Could you check a few things on this drawing? It's one solid part, dimensions in mm from its lowest x, y, z. Give positions to 0.01 mm unless a question says otherwise; leave off trailing zeros. Write each loop counter-clockwise with the first axis right and the second up, starting at its lowest first coordinate (ties: lowest second). Pieces come first, ordered by that corner, then holes. Notation, with made-up numbers: (49.5, 45.5) -> (72.5, 45.5) arc R19 ccw to (72.5, 80.5) -> close; hole circle Ø8 at (10.25, 75.5). An arc over 180 degrees is marked (long way). Answer as CSV lines item,"result". Start each with the question number.
1. If we section it at D-D on z = 8.5: Write out the boundary of the cut face in (x, y) (1 decimal), plus the area to 3 significant figures.
2. I'm going to push flat-ended pins straight in: P1, Ø1.5, axis at x = 18.5, y = 2.5, coming from the +Z side; P2, Ø1.5, axis at x = 14.5, y = 2, coming from the -Z side. Where does each tip first touch, or does it pass through?
3. If we section it at B-B on z = 34: Write out the boundary of the cut face in (x, y) (1 decimal).
4. I need wall thicknesses on line 1 (X direction, y = 1.75, z = 18.5) (1 decimal); line 2 (X direction, y = 4.45, z = 32); line 3 (Y direction, x = 3.5, z = 32.5) (1 decimal). Which ranges of each line are inside material? Lowest first, please. Write a range as [from, to].
5. If we mould it in two halves opening along X, with no side actions, what happens to the marked faces 1, 2, 3 and 4? For each: pulls with the +X half, pulls with the -X half, needs draft (parallel to the pull), parting line crosses it, or undercut.
6. If we section it at A-A on y = 2.5: Count the separate pieces of the cut face and the enclosed holes in it.
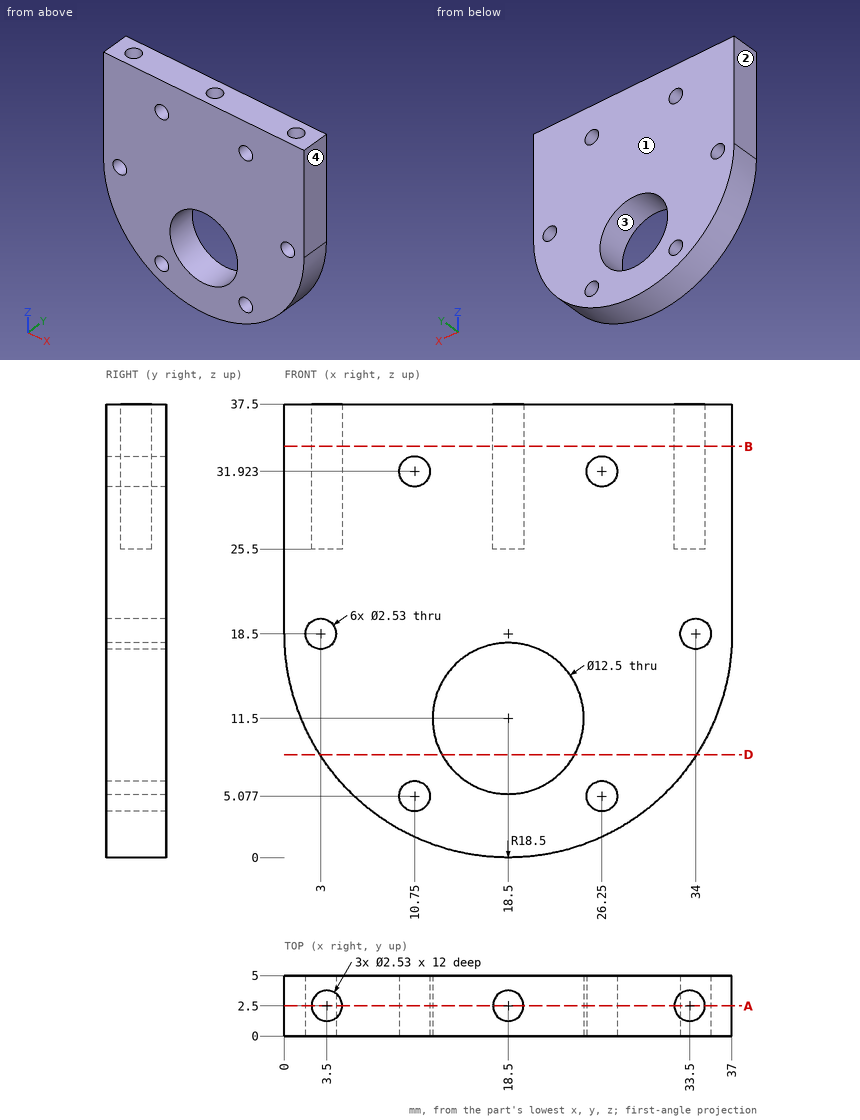
Computed values:
1,outline,"(2.9, 0) -> (13, 0) -> (13, 5) -> (2.9, 5) -> close; (24, 0) -> (34.1, 0) -> (34.1, 5) -> (24, 5) -> close"
1,area,"101 mm2"
2,P1,"stops at z = 25.5"
2,P2,"stops at z = 0.29"
3,outline,"(0, 0) -> (37, 0) -> (37, 5) -> (0, 5) -> close; hole circle Ø2.5 at (3.5, 2.5); hole circle Ø2.5 at (18.5, 2.5); hole circle Ø2.5 at (33.5, 2.5)"
4,line 1,"x = [0, 1.7], [4.3, 32.7], [35.3, 37]"
4,line 2,"x = [0, 9.49], [12.01, 24.99], [27.51, 37]"
4,line 3,"y = [0, 1.2], [3.8, 5]"
5,face 1,"needs draft"
5,face 2,"pulls with the -X half"
5,face 3,"undercut"
5,face 4,"pulls with the +X half"
6,separate pieces,"1"
6,enclosed holes,"7"
